Could you check a few things on this model? Use its own coordinates, in mm. Coordinates: 2 decimals unless noted, no trailing zeros. Write each loop counter-clockwise with the first axis right and the second up, starting at its lowest first coordinate (ties: lowest second). Pieces come first, ordered by that corner, then holes.
```python
from build123d import *

# Parameters (mm, degrees)
SKETCH1_W               = 95.25
SKETCH1_H               = 50.8
BOSS_EXTRUDE1_DEPTH     = 3
CUT_EXTRUDE1_DEPTH      = 55.058307641
CUT_EXTRUDE1_DEPTH_BACK = 55.058307641
SKETCH2_R               = 21.75


with BuildPart() as part:
    # Sketch1 → Boss-Extrude1 (new body)
    with BuildSketch(Plane(origin=(0, 0, 0), x_dir=(1, 0, 0), z_dir=(0, 1, 0))):
        Rectangle(SKETCH1_W, SKETCH1_H)
    extrude(amount=BOSS_EXTRUDE1_DEPTH)

    # Sketch2 → Cut-Extrude1 (cut, two sides: drawn at the far end of the back side and taken through both)
    with BuildSketch(Plane(origin=(0, 3, 0), x_dir=(1, 0, 0), z_dir=(0, 1, 0)).offset(-CUT_EXTRUDE1_DEPTH_BACK)):
        with Locations(Location((0, 0, 0), (0, 0, 270))):
            Circle(SKETCH2_R)
    extrude(amount=CUT_EXTRUDE1_DEPTH + CUT_EXTRUDE1_DEPTH_BACK, mode=Mode.SUBTRACT)


solid = part.part
```
1. If we mould it in two halves opening along Z, with no side actions, what happens to faces 1 (the face through (-22, 3, 0)), 2 (the face through (-1, 1, -25.4)), 3 (the face through (21.565, 1.479, -2.831))? For each: pulls with the +Z half, pulls with the -Z half, needs draft (parallel to the pull), parting line crosses it, or undercut.
Verdict:
face 1: needs draft
face 2: pulls with the -Z half
face 3: undercut
2. I want a section at A-A on x = 0. Please give me the cut outline in (y, z).
Verdict:
outline: (0, -25.4) - (3, -25.4) - (3, -21.75) - (0, -21.75) - close; (0, 21.75) - (3, 21.75) - (3, 25.4) - (0, 25.4) - close
3. I want a section at B-B on z = 0. Please give me the cut outline in (x, y) (3 decimals).
Verdict:
outline: (-47.625, 0) - (-21.75, 0) - (-21.75, 3) - (-47.625, 3) - close; (21.75, 0) - (47.625, 0) - (47.625, 3) - (21.75, 3) - close
4. For pin 1 (6 mm diameter, centred on x = -18, z = 6.5, fed in from +Y), with a flat end and sliding along its axis, tell me the tip position at first contact or that it passes through.
Verdict:
pin 1: stops at y = 3
5. I want a section at C-C on y = 1.6. Please give me the cut outline in (x, z) (3 decimals), plus the area to 3 significant figures.
Verdict:
outline: (-47.625, -25.4) - (47.625, -25.4) - (47.625, 25.4) - (-47.625, 25.4) - close; hole circle Ø43.5 at (0, 0)
area: 3,350 mm2
6. Please list where these lines run through material, in increasing order: line 1 along Z through (x, y) = (0, 0.9); line 2 along X through (y, z) = (1.9, 0) (3 decimals); line 3 along X through (y, z) = (2.55, -19) (3 decimals).
Verdict:
line 1: z = -25.4 to -21.75, 21.75 to 25.4
line 2: x = -47.625 to -21.75, 21.75 to 47.625
line 3: x = -47.625 to -10.586, 10.586 to 47.625
